```python
from build123d import *

# Parameters (mm, degrees)
F2_R = 10
F3_R = 30


with BuildPart() as f1:
    # F0 (on Front) → F1 (revolve)
    with BuildSketch(Plane.XZ):
        Polygon((0, 1650), (-150, 1650), (-225, 1176.468636), (-75, 1176.468636), (-69.710191, 1146.468636), (-190.2089, 0), (0, 0), align=None)
    revolve(axis=Axis((0, 0, 825), (0, 0, 1)))

    # F2
    f2_edges = [f1.edges().sort_by_distance(p)[0] for p in [
        (150, 0, 1650),
        (225, 0, 1176.468636),
        (190.2089, 0, 0),
    ]]
    fillet(f2_edges, radius=F2_R)

    # F3
    f3_edges = [f1.edges().sort_by_distance(p)[0] for p in [
        (75, 0, 1176.468636),
        (69.710191, 0, 1146.468636),
    ]]
    fillet(f3_edges, radius=F3_R)


solid = f1.part
```
Input: part model. Units: mm. Frame: model coordinates. A direction names the side the tool comes from. Give positions to 0.01 mm unless a question says otherwise; leave off trailing zeros. Order: outer loops, then holes, each group sorted by start corner. A loop starts at its lowest first (then second) coordinate and runs counter-clockwise, first axis right, second up. Notation, with made-up numbers: (9.5, 6) - (32.5, 6) arc R25 ccw to (32.5, 44) - close; hole circle Ø9 at (57.25, 33). An arc over 180 degrees is marked (long way). One line per item, written item: value.
1. Cut plane A-A, the plane z = 716. Output: boundary loops of the cut face in (x, y).
Determined:
outline: circle Ø229.91 at (0, 0)
2. Pin query (flat end, axial travel): pin 1 Ø8 at (y, z) = (105, 382) entering from +X; pin 2 Ø6 at (y, z) = (97.5, 618) entering from +X; pin 3 Ø4 at (y, z) = (130, 1320) entering from -X. Return the tip coordinate at first contact, or that it passes through.
Determined:
pin 1: x = 111.02
pin 2: x = 82.24
pin 3: x = -156.66
3. Line query: probe 1 along X at (y, z) = (11.5, 906); probe 2 along Y at (x, z) = (-42.5, 1082); probe 3 along X at (y, z) = (121, 235.5). Output: solid intervals per line, ascending.
Determined:
probe 1: -94.29 to 94.29
probe 2: -63.59 to 63.59
probe 3: -112.85 to 112.85
4. Draft query along Z for faces 1 (the face through (-2, -2, 1650)), 2 (the face through (3, -3, 0)), 3 (the face through (-44, 92, 1176.469)). Return one class per face: released by +Z, released by -Z, zero draft, split by the parting line, or undercut.
Determined:
face 1: released by +Z
face 2: released by -Z
face 3: undercut
5. Reachability of faces 4 (the face through (-171.47, -54, 1462.02)), 5 (the face through (-124.41, -39.18, 568.74)) from +Z, -Z, +X, -X, +Y, -Y: full face, straight path, thin tool, end or side. Return the list, or none.
Determined:
face 4: +Z
face 5: none
6. Cut plane B-B, the plane z = 1016. Output: boundary loops of the cut face in (x, y), and give its area (3 significant figures).
Determined:
outline: circle Ø166.85 at (0, 0)
area: 21,900 mm2
